Design review of the part shown in the three views and the two pictorial views. Dimensions are in mm from the part's minimum x, y and z. Give positions to 0.01 mm unless a question says otherwise; leave off trailing zeros. Order: outer loops, then holes, each group sorted by start corner. A loop starts at its lowest first (then second) coordinate and runs counter-clockwise, first axis right, second up.
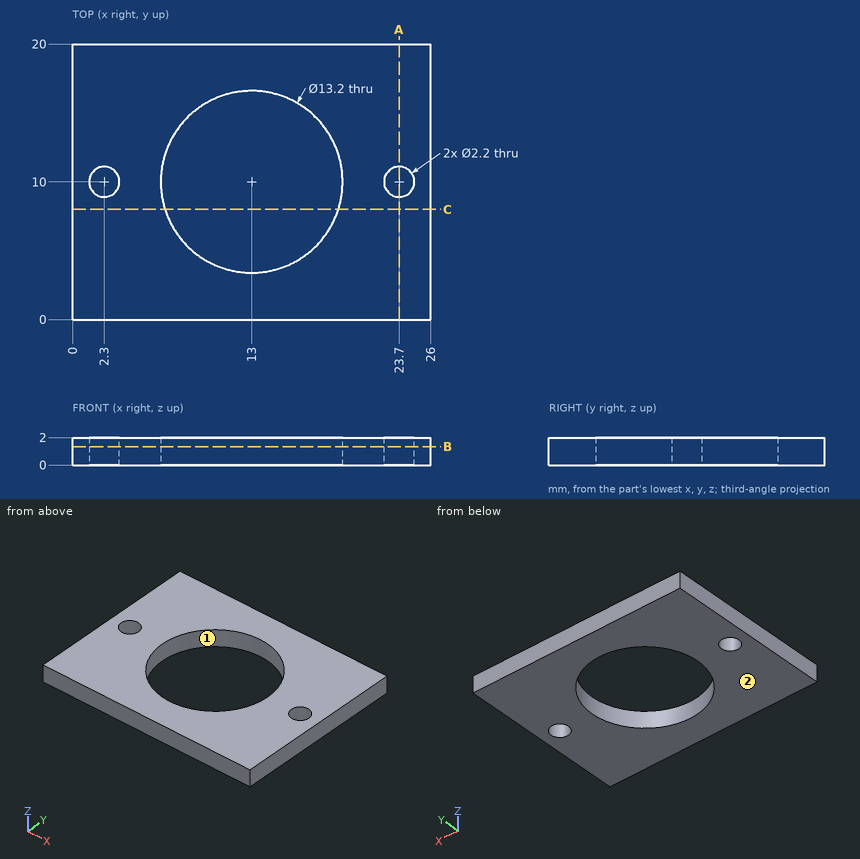
1) Clearance check with flat-ended pins moving along their axes: pin 1 (1.8 mm diameter, centred on x = 23.7, y = 10, fed in from +Z); pin 2 (3.5 mm diameter, centred on x = 2.3, y = 10, fed in from -Z). State where each tip first meets the part, or that it passes through.
Answer sheet:
pin 1: passes through
pin 2: stops at z = 0
2) Draft analysis for pull direction X (two halves, no side actions). For the marked faces 1 and 2, state which applies: +X half, -X half, draft (parallel to the pull), parting line (faces both ways), or undercut.
Answer sheet:
face 1: undercut
face 2: draft
3) We need section A-A on x = 23.7. Give the boundary of the cut face in (y, z), then the cut area to 3 significant figures.
Answer sheet:
outline: (0, 0) - (8.9, 0) - (8.9, 2) - (0, 2) - close; (11.1, 0) - (20, 0) - (20, 2) - (11.1, 2) - close
area: 35.6 mm2
4) We need section C-C on y = 8. Give the boundary of the cut face in (x, z), then the cut area to 3 significant figures.
Answer sheet:
outline: (0, 0) - (6.71, 0) - (6.71, 2) - (0, 2) - close; (19.29, 0) - (26, 0) - (26, 2) - (19.29, 2) - close
area: 26.8 mm2
5) We need section B-B on z = 1.35. Give the boundary of the cut face in (x, y), then the cut area to 3 significant figures.
Answer sheet:
outline: (0, 0) - (26, 0) - (26, 20) - (0, 20) - close; hole circle Ø2.2 at (2.3, 10); hole circle Ø13.2 at (13, 10); hole circle Ø2.2 at (23.7, 10)
area: 376 mm2
6) To check wall thickness, follow line 1 (Y direction, x = 13, z = 0.55); line 2 (Y direction, x = 23.7, z = 1.05); line 3 (X direction, y = 9.75, z = 1.55). State the ranges of each line that lie inside material, in increasing order.
Answer sheet:
line 1: y = 0 to 3.4, 16.6 to 20
line 2: y = 0 to 8.9, 11.1 to 20
line 3: x = 0 to 1.23, 3.37 to 6.4, 19.6 to 22.63, 24.77 to 26
